from build123d import *

# Parameters (mm, degrees)
PAD_DEPTH = 65


with BuildPart() as part:
    # Sketch → Pad (new body)
    with BuildSketch(Plane.XY):
        with BuildLine():
            ThreePointArc((18.116844, 13.5), (0, 9.5), (18.116844, 5.5))
            Line((18.116844, 5.5), (19.883156, 5.5))
            ThreePointArc((19.883156, 5.5), (28.5, 0), (37.116844, 5.5))
            Line((37.116844, 5.5), (38.883156, 5.5))
            ThreePointArc((38.883156, 5.5), (47.5, 0), (56.116844, 5.5))
            Line((56.116844, 5.5), (57.883156, 5.5))
            ThreePointArc((57.883156, 5.5), (76, 9.5), (57.883156, 13.5))
            Line((57.883156, 13.5), (56.116844, 13.5))
            ThreePointArc((56.116844, 13.5), (47.5, 19), (38.883156, 13.5))
            Line((38.883156, 13.5), (37.116844, 13.5))
            ThreePointArc((37.116844, 13.5), (28.5, 19), (19.883156, 13.5))
            Line((19.883156, 13.5), (18.116844, 13.5))
        make_face()
    extrude(amount=PAD_DEPTH)


solid = part.part
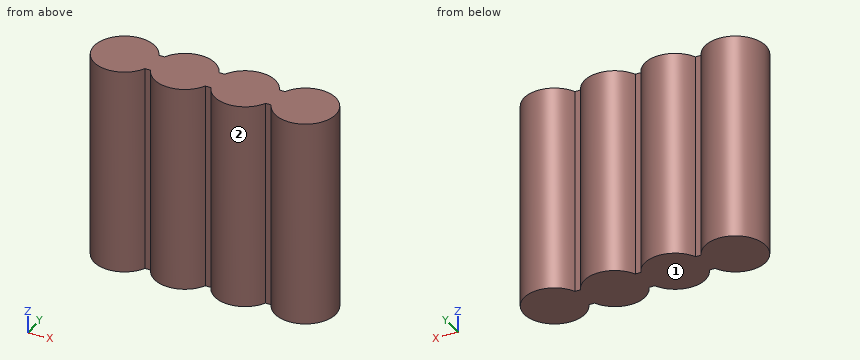
Could you check a few things on this model? Use its own coordinates, in mm. Face numbers are marked on the shaded views. Give positions to 0.01 mm unless a question says otherwise; leave off trailing zeros. Order: outer loops, then holes, each group sorted by start corner. A loop starts at its lowest first (then second) coordinate and runs counter-clockwise, first axis right, second up. Notation, with made-up numbers: (-13, -33.5) - (1, -33.5) arc R23 cw to (1, -0.5) - close; hole circle Ø9 at (46, 13). An arc over 180 degrees is marked (long way). One line per item, written item: value. Start each with the question number.
1. Imagine slicing it at A-A on z = 20. List the corners of the cut face in (x, y) for me, plus the area to 3 significant figures.
2. Thinking about a two-plate mould opening in X: for the marked faces 1 and 2, which applies, +X half, -X half, draft (parallel to the pull), parting line (faces both ways), or undercut?
3. Imagine slicing it at B-B on x = 26. List the corners of the cut face in (y, z) for me.
4. For P1, Ø3, axis at y = 4.5, z = 56.5, coming from the +X side; P2, Ø10, axis at x = 56.5, y = 4, coming from the +Z side; P3, Ø4, axis at x = 19.5, z = 11, coming from the +Y side; P4, Ø1.4, axis at x = 38, z = 23, coming from the +Y side, each with a flat end and sliding along its axis, tell me the tip position at first contact or that it passes through.
5. If I drill on probe 1 along X at (y, z) = (15, 8); probe 2 along X at (y, z) = (4.5, 28); probe 3 along Y at (x, z) = (47, 33), over which ranges is the centre line in solid material (lowest first)?
6. Imagine slicing it at C-C on x = 14. List the corners of the cut face in (y, z) for me.
Values:
1. outline: (18.12, 5.5) - (19.88, 5.5) arc R9.5 ccw to (37.12, 5.5) - (38.88, 5.5) arc R9.5 ccw to (56.12, 5.5) - (57.88, 5.5) arc R9.5 ccw (long way) to (57.88, 13.5) - (56.12, 13.5) arc R9.5 ccw to (38.88, 13.5) - (37.12, 13.5) arc R9.5 ccw to (19.88, 13.5) - (18.12, 13.5) arc R9.5 ccw (long way) to start
1. area: 1,150 mm²
2. face 1: draft
2. face 2: undercut
3. outline: (0.33, 0) - (18.67, 0) - (18.67, 65) - (0.33, 65) - close
4. P1: x = 75.33
4. P2: z = 65
4. P3: y = 15.92
4. P4: y = 13.5
5. probe 1: 1.75 to 17.25, 20.75 to 36.25, 39.75 to 55.25, 58.75 to 74.25
5. probe 2: 1.42 to 17.58, 20.42 to 36.58, 39.42 to 55.58, 58.42 to 74.58
5. probe 3: 0.01 to 18.99
6. outline: (1.13, 0) - (17.87, 0) - (17.87, 65) - (1.13, 65) - close
